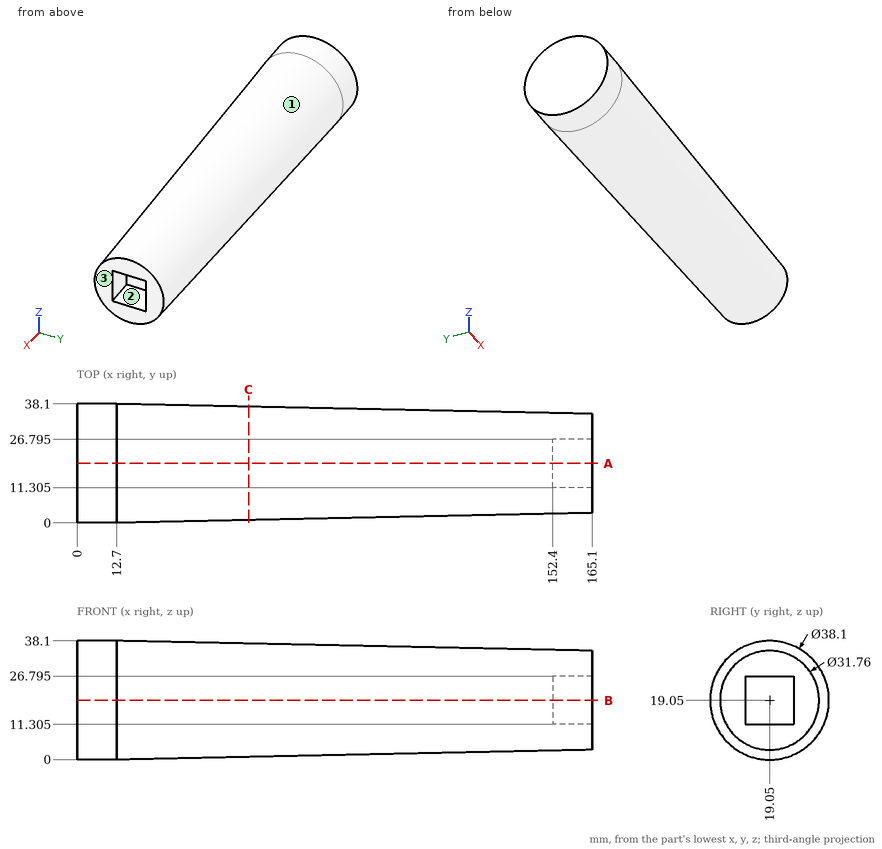
Check sheet for the drawn part. Datum: minimum x, y, z corner. Units: mm. Give positions to 0.01 mm unless a question says otherwise; leave off trailing zeros. Order: outer loops, then holes, each group sorted by start corner. A loop starts at its lowest first (then second) coordinate and runs counter-clockwise, first axis right, second up. Notation, with made-up numbers: (-15.5, 74) - (-6.5, 74) arc R20 cw to (-6.5, 113) - close; hole circle Ø4 at (32.25, -12). An arc over 180 degrees is marked (long way). Answer in a Markdown table with one row per item. Add a question column.
Q1. Cross-section at A-A, the plane y = 19.05. Enter the section's corners in (x, z) (3 decimals).
Q2. Gauge pin test, flat ends, axial feed: pin 1 (4.5 mm diameter, centred on y = 19, z = 16.5, fed in from +X); pin 2 (5 mm diameter, centred on x = 45, z = 15, fed in from -Y); pin 3 (6.5 mm diameter, centred on x = 161, y = 16.5, fed in from +Z). Record the tip position at first contact, or that the pin passes through.
Q3. Cross-section at C-C, the plane x = 55. Enter the section's corners in (y, z).
Q4. Mould release check, pull along Z, two halves, no side actions. Record for the marked faces 1, 2 and 3: pulls with the +Z half, pulls with the -Z half, needs draft (parallel to the pull), parting line crosses it, or undercut.
Q5. Material ranges on probe 1 along X at (y, z) = (16, 26.5); probe 2 along Y at (x, z) = (87, 12); probe 3 along Z at (x, y) = (14.5, 22), recorded low to high. Write a range as from..to.
Check values:
| question | item | result |
|---|---|---|
| 1 | outline | (0, 0) - (12.7, 0) - (165.1, 3.17) - (165.1, 11.305) - (152.4, 11.305) - (152.4, 26.795) - (165.1, 26.795) - (165.1, 34.93) - (12.7, 38.1) - (0, 38.1) - close |
| 2 | pin 1 | stops at x = 152.4 |
| 2 | pin 2 | stops at y = 0.73 |
| 2 | pin 3 | stops at z = 35.06 |
| 3 | outline | circle Ø36.34 at (19.05, 19.05) |
| 4 | face 1 | parting line crosses it |
| 4 | face 2 | undercut |
| 4 | face 3 | needs draft |
| 5 | probe 1 | x = 0..152.4 |
| 5 | probe 2 | y = 3.03..35.07 |
| 5 | probe 3 | z = 0.27..37.83 |
